CAD build for the part. Positions are in the model's coordinates, mm. Face numbers are marked on the shaded views. A direction names the side the tool comes from. Round coordinates to 2 decimals unless told otherwise and drop trailing zeros. Loops run counter-clockwise (first coordinate to the right, second up) from the corner with the lowest first, then second, coordinate; pieces in that order, holes last. Notation, with made-up numbers: M 49.25,16 L 94.25,16 A30 ccw 94.25,40 Z; hole C 55.25,-1.75 d5. An arc over 180 degrees is marked long. Use a Markdown table: item, result. Add a question column.
(1) Flat gauge pins, fed straight in: P1, Ø4, axis at x = 85.5, y = 47.5, coming from the -Z side; P2, Ø3, axis at x = 71, y = 167.5, coming from the +Z side; P3, Ø12, axis at y = 60.5, z = 318.5, coming from the +X side; P4, Ø5.5, axis at x = 33, z = 257, coming from the +Y side. Where does each tip first touch, or does it go through?
(2) Two-plate mould, pull along X, no slides. Class the marked faces 1, 2 and 3: released by +X, released by -X, zero draft, split by the parting line, or undercut.
(3) Wall check: L1, parallel to Y at x = 66.5, z = 179; L2, parallel to X at y = -4.5, z = 175; L3, parallel to X at y = 129.5, z = 123.5. Give the ranges that are in metal, low to high.
(4) Band-saw the part on B-B, the plane y = 36. Write the cut outline in (x, z).
(5) Band-saw the part on C-C, the plane z = 249. Write the cut outline in (x, y).
(6) Which spindle directions (+Z, -Z, +X, -X, +Y, -Y) get a long thin tool onto all of the face, cutting with end or side? Do the marked faces 4, 5 and 6. Say none if no direction does.
(7) Band-saw the part on D-D, the plane z = 346. Write the cut outline in (x, y), and give its area (3 significant figures).
(8) Band-saw the part on A-A, the plane x = 67. Write the cut outline in (y, z).
from build123d import *

# Parameters (mm, degrees)
CROQUIS1_W              = 150
CROQUIS1_H              = 200
SALIENTE_EXTRUIR1_DEPTH = 200
VACIADO1_T              = -3
CROQUIS2_R              = 10
SALIENTE_EXTRUIR2_DEPTH = 100
CROQUIS3_R              = 12.7
SALIENTE_EXTRUIR3_DEPTH = 3
CROQUIS6_R              = 5
SALIENTE_EXTRUIR4_DEPTH = 5
SALIENTE_EXTRUIR5_START = -5
CROQUIS8_R              = 5
SALIENTE_EXTRUIR5_DEPTH = 5


with BuildPart() as part:
    # Croquis1 → Saliente-Extruir1 (new body)
    with BuildSketch(Plane.XY):
        with Locations((75, 100)):
            Rectangle(CROQUIS1_W, CROQUIS1_H)
    extrude(amount=SALIENTE_EXTRUIR1_DEPTH)

    # Vaciado1
    vaciado1_openings = [part.faces().sort_by_distance(p)[0] for p in [
        (75, 100, 200),
    ]]
    offset(amount=VACIADO1_T, openings=vaciado1_openings, kind=Kind.INTERSECTION)

    # Croquis2 → Saliente-Extruir2 (add)
    with BuildSketch(Plane.ZY.offset(-147)):
        with Locations((33, 100)):
            Circle(CROQUIS2_R)
        with Locations((180, 180)):
            Circle(CROQUIS2_R)
        with Locations(Location((180, 20, 0), (0, 0, 180))):
            Circle(CROQUIS2_R)
    extrude(amount=SALIENTE_EXTRUIR2_DEPTH)

    # Croquis3 → Saliente-Extruir3 (add)
    with BuildSketch(Plane(origin=(150, 0, 0), x_dir=(0, 0, -1), z_dir=(1, 0, 0))):
        with BuildLine():
            Line((-371.678920241, 124.009678041), (0, 150))
            Line((0, 150), (0, 50))
            Line((0, 50), (-371.678920241, 75.990321959))
            ThreePointArc((-371.678920241, 75.990321959), (-394.068307228, 100), (-371.678920241, 124.009678041))
        make_face()
        with Locations((-370, 100)):
            Circle(CROQUIS3_R, mode=Mode.SUBTRACT)
    saliente_extruir3 = extrude(amount=SALIENTE_EXTRUIR3_DEPTH)

    # Simetría1: Saliente-Extruir3 across plane
    add(saliente_extruir3.mirror(Plane(origin=(75, 0, 0), x_dir=(0, 0, 1), z_dir=(1, 0, 0))))

    # Croquis6 → Saliente-Extruir4 (add)
    with BuildSketch(Plane(origin=(30, 0, 0), x_dir=(0, 0, -1), z_dir=(1, 0, 0))):
        with BuildLine():
            Line((-200, 0), (-200, -66.865061558))
            Line((-200, -66.865061558), (-325, -66.865061558))
            ThreePointArc((-325, -66.865061558), (-335, -76.865061558), (-325, -86.865061558))
            Line((-325, -86.865061558), (-170, -86.865061558))
            Line((-170, -86.865061558), (-170, 0))
            Line((-170, 0), (-200, 0))
        make_face()
        with Locations((-325, -76.865061558)):
            Circle(CROQUIS6_R, mode=Mode.SUBTRACT)
        with Locations((-260, -76.865061558)):
            Circle(CROQUIS6_R, mode=Mode.SUBTRACT)
    extrude(amount=SALIENTE_EXTRUIR4_DEPTH)

    # Croquis8 → Saliente-Extruir5 (add)
    with BuildSketch(Plane(origin=(150, 0, 0), x_dir=(0, 0, -1), z_dir=(1, 0, 0)).offset(SALIENTE_EXTRUIR5_START)):
        with BuildLine():
            Line((-200, -66.865061558), (-325, -66.865061558))
            ThreePointArc((-325, -66.865061558), (-335, -76.865061558), (-325, -86.865061558))
            Line((-325, -86.865061558), (-170, -86.865061558))
            Line((-170, -86.865061558), (-170, 0))
            Line((-170, 0), (-200, 0))
            Line((-200, 0), (-200, -66.865061558))
        make_face()
        with Locations((-260, -76.865061558)):
            Circle(CROQUIS8_R, mode=Mode.SUBTRACT)
        with Locations((-325, -76.865061558)):
            Circle(CROQUIS8_R, mode=Mode.SUBTRACT)
    extrude(amount=SALIENTE_EXTRUIR5_DEPTH)


solid = part.part
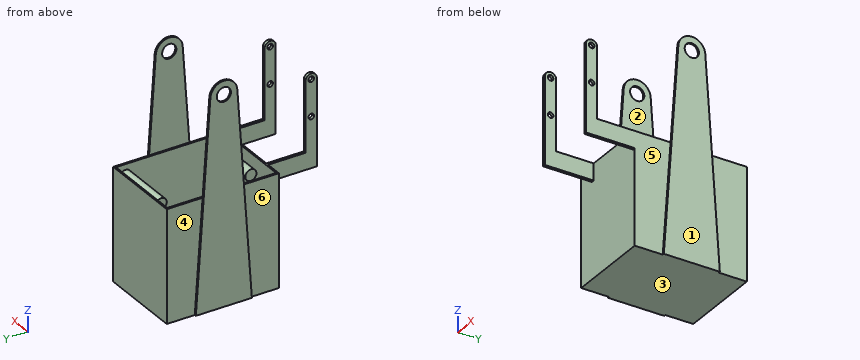
Return value:
| question | item | result |
|---|---|---|
| 1 | P1 | z = 0 |
| 1 | P2 | z = 3 |
| 1 | P3 | through |
| 1 | P4 | y = -66.87 |
| 2 | face 1 | released by +X |
| 2 | face 2 | undercut |
| 2 | face 3 | zero draft |
| 3 | L1 | 0 to 3, 10.05 to 29.95, 170.05 to 189.95, 197 to 200 |
| 3 | L2 | 30 to 35, 145 to 150 |
| 3 | L3 | -3 to 3, 147 to 153 |
| 4 | outline | M 0,0 L 150,0 L 150,200 L 147,200 L 147,3 L 3,3 L 3,200 L 0,200 Z |
| 5 | outline | M -3,67.41 L 0,67.41 L 0,132.59 L -3,132.59 Z; M 30,-86.87 L 35,-86.87 L 35,-66.87 L 30,-66.87 Z; M 145,-86.87 L 150,-86.87 L 150,-66.87 L 145,-66.87 Z; M 150,67.41 L 153,67.41 L 153,132.59 L 150,132.59 Z |
| 6 | face 4 | +Z, -X, +Y |
| 6 | face 5 | +Z, +X, -Y |
| 6 | face 6 | +Z, -X, -Y |
| 7 | outline | M -3,74.19 L 0,74.19 L 0,125.81 L -3,125.81 Z; M 150,74.19 L 153,74.19 L 153,125.81 L 150,125.81 Z |
| 7 | area | 310 mm^2 |
| 8 | outline | M 0,0 L 200,0 L 200,200 L 197,200 L 197,3 L 3,3 L 3,200 L 0,200 Z; C 20,180 d20; C 100,33 d20; C 180,180 d20 |
